Geometry check sheet. Reference: the model listing, model coordinates, mm. Face numbers are marked on the shaded views. A direction names the side the tool comes from. Coordinates: 2 decimals unless noted, no trailing zeros. Loops run counter-clockwise (first coordinate to the right, second up) from the corner with the lowest first, then second, coordinate; pieces in that order, holes last. Notation, with made-up numbers: (72.5, 80) -> (125.5, 80) arc R5 cw to (125.5, 84) -> close; hole circle Ø10 at (-14.75, -25.5). An arc over 180 degrees is marked (long way). Answer as a JSON object with one key per item and string values.
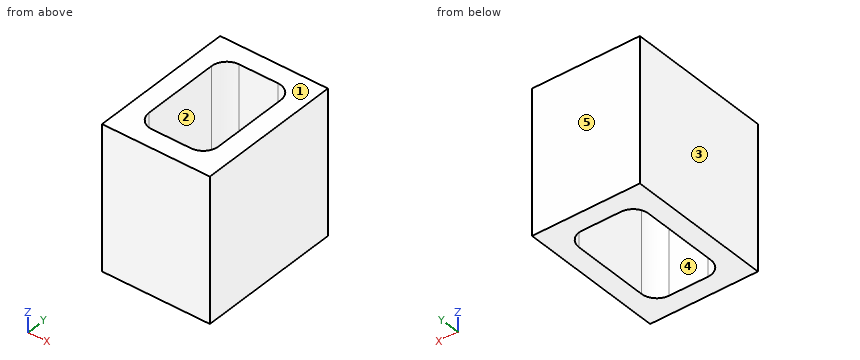
from build123d import *

# Parameters (mm, degrees)
F0_W     = 142.875
F0_H     = 193.675
F1_DEPTH = 95.25


with BuildPart() as f1:
    # F0 (on Top) → F1 (new body, symmetric)
    with BuildSketch(Plane.XY):
        Rectangle(F0_W, F0_H)
        with BuildLine():
            Line((-25.7175, 71.4375), (25.7175, 71.4375))
            ThreePointArc((25.7175, 71.4375), (40.08591, 65.48591), (46.0375, 51.1175))
            Line((46.0375, 51.1175), (46.0375, 0))
            Line((46.0375, 0), (46.0375, -51.1175))
            ThreePointArc((46.0375, -51.1175), (40.08591, -65.48591), (25.7175, -71.4375))
            Line((25.7175, -71.4375), (-25.7175, -71.4375))
            ThreePointArc((-25.7175, -71.4375), (-40.08591, -65.48591), (-46.0375, -51.1175))
            Line((-46.0375, -51.1175), (-46.0375, 0))
            Line((-46.0375, 0), (-46.0375, 51.1175))
            ThreePointArc((-46.0375, 51.1175), (-40.08591, 65.48591), (-25.7175, 71.4375))
        make_face(mode=Mode.SUBTRACT)
    extrude(amount=F1_DEPTH, both=True)


solid = f1.part
1. Thickness scan on probe 1 along X at (y, z) = (-31.5, -16.5); probe 2 along Y at (x, z) = (-11.5, -2); probe 3 along X at (y, z) = (-65, -40). Record the ranges inside material, lowest first. Write a range as from..to.
Evaluation:
{"probe 1": "x = -71.44..-46.04, 46.04..71.44", "probe 2": "y = -96.84..-71.44, 71.44..96.84", "probe 3": "x = -71.44..-40.56, 40.56..71.44"}
2. Section check C-C, the plane z = -42. Record the boundary of the cut face in (x, y), then the cut area to 3 significant figures.
Evaluation:
{"outline": "(-71.44, -96.84) -> (71.44, -96.84) -> (71.44, 96.84) -> (-71.44, 96.84) -> close; hole (-46.04, -51.12) arc R20.32 ccw to (-25.72, -71.44) -> (25.72, -71.44) arc R20.32 ccw to (46.04, -51.12) -> (46.04, 51.12) arc R20.32 ccw to (25.72, 71.44) -> (-25.72, 71.44) arc R20.32 ccw to (-46.04, 51.12) -> close", "area": "14,900 mm^2"}
3. Tool access check on the marked faces 1 and 2. Record the directions out of +Z, -Z, +X, -X, +Y, -Y that give a thin tool (end or side, any length) a straight path to the whole face; none if there is none.
Evaluation:
{"face 1": "+Z, +X, -X, +Y, -Y", "face 2": "+Z, -Z"}
4. Section check A-A, the plane y = 27. Record the boundary of the cut face in (x, z).
Evaluation:
{"outline": "(-71.44, -95.25) -> (-46.04, -95.25) -> (-46.04, 95.25) -> (-71.44, 95.25) -> close; (46.04, -95.25) -> (71.44, -95.25) -> (71.44, 95.25) -> (46.04, 95.25) -> close"}
5. Section check B-B, the plane x = -19.5. Record the boundary of the cut face in (y, z).
Evaluation:
{"outline": "(-96.84, -95.25) -> (-71.44, -95.25) -> (-71.44, 95.25) -> (-96.84, 95.25) -> close; (71.44, -95.25) -> (96.84, -95.25) -> (96.84, 95.25) -> (71.44, 95.25) -> close"}
6. Mould release check, pull along X, two halves, no side actions. Record for the marked faces 3, 4 and 5: released by +X, released by -X, zero draft, split by the parting line, or undercut.
Evaluation:
{"face 3": "released by -X", "face 4": "undercut", "face 5": "zero draft"}
7. Depth check by flat-ended pin: P1, Ø8, axis at x = 41.5, y = -10, coming from the -Z side. Enter the tip coordinate at first touch or a pass-through.
Evaluation:
{"P1": "passes through"}
